from build123d import *

# Parameters (mm, degrees)
SKETCH_1_W          = 52
SKETCH_1_H          = 63
EXTRUDE_1_DEPTH     = 8
SKETCH_2_W          = 48.4
SKETCH_2_H          = 59.4
CUT_EXTRUDE_1_DEPTH = 6.3
FILLET_1_R          = 2
CUT_EXTRUDE_2_REACH = 43.327
SKETCH_3_R          = 3.2
CUT_EXTRUDE_3_REACH = 43.327
SKETCH_4_R          = 18
SKETCH_4_W          = 13.4
SKETCH_4_H          = 3
CUT_EXTRUDE_4_REACH = 43.327
SKETCH_5_W          = 5.3
SKETCH_5_H          = 3.2
SKETCH_6_W          = 10
SKETCH_6_H          = 2.2
SKETCH_6_W_2        = 4.8
SKETCH_6_W_3        = 6.5
SKETCH_6_H_2        = 10
CUT_EXTRUDE_5_DEPTH = 1
CUT_EXTRUDE_6_REACH = 61.802
SKETCH_7_W          = 6.3
SKETCH_7_H          = 10


with BuildPart() as part:
    # 草图1 → 凸台-拉伸1 (new body)
    with BuildSketch(Plane.XY):
        Rectangle(SKETCH_1_W, SKETCH_1_H)
    extrude(amount=EXTRUDE_1_DEPTH)

    # 草图2 → 切除-拉伸1 (cut)
    with BuildSketch(Plane.XY.offset(8)):
        Rectangle(SKETCH_2_W, SKETCH_2_H)
    extrude(amount=-CUT_EXTRUDE_1_DEPTH, mode=Mode.SUBTRACT)

    # 圆角1
    fillet_1_edges = [part.edges().sort_by_distance(p)[0] for p in [
        (26, -31.5, 4),
        (-26, -31.5, 4),
        (-26, 31.5, 4),
        (26, 31.5, 4),
    ]]
    fillet(fillet_1_edges, radius=FILLET_1_R)

    # 草图3 → 切除-拉伸2 (cut, up to next)
    with BuildSketch(Plane.XY.offset(1.7), mode=Mode.PRIVATE) as cut_extrude_2_sk1:
        with Locations((0, 24)):
            Circle(SKETCH_3_R)
    cut_extrude_2_tool1 = extrude(cut_extrude_2_sk1.sketch, amount=-CUT_EXTRUDE_2_REACH, mode=Mode.PRIVATE) & part.part
    # 草图3 → 切除-拉伸2 (cut, up to next)
    with BuildSketch(Plane.XY.offset(1.7), mode=Mode.PRIVATE) as cut_extrude_2_sk2:
        with Locations((-17.8, -24)):
            Circle(SKETCH_3_R)
    cut_extrude_2_tool2 = extrude(cut_extrude_2_sk2.sketch, amount=-CUT_EXTRUDE_2_REACH, mode=Mode.PRIVATE) & part.part
    # 草图3 → 切除-拉伸2 (cut, up to next)
    with BuildSketch(Plane.XY.offset(1.7), mode=Mode.PRIVATE) as cut_extrude_2_sk3:
        with Locations((17.8, -24)):
            Circle(SKETCH_3_R)
    cut_extrude_2_tool3 = extrude(cut_extrude_2_sk3.sketch, amount=-CUT_EXTRUDE_2_REACH, mode=Mode.PRIVATE) & part.part
    add(cut_extrude_2_tool1.solids().sort_by_distance((0, 24, 1.7))[0], mode=Mode.SUBTRACT)
    add(cut_extrude_2_tool2.solids().sort_by_distance((-17.8, -24, 1.7))[0], mode=Mode.SUBTRACT)
    add(cut_extrude_2_tool3.solids().sort_by_distance((17.8, -24, 1.7))[0], mode=Mode.SUBTRACT)

    # 草图4 → 切除-拉伸3 (cut, up to next)
    with BuildSketch(Plane.XY.offset(1.7), mode=Mode.PRIVATE) as cut_extrude_3_sk1:
        Circle(SKETCH_4_R)
    cut_extrude_3_tool1 = extrude(cut_extrude_3_sk1.sketch, amount=-CUT_EXTRUDE_3_REACH, mode=Mode.PRIVATE) & part.part
    # 草图4 → 切除-拉伸3 (cut, up to next)
    with BuildSketch(Plane.XY.offset(1.7), mode=Mode.PRIVATE) as cut_extrude_3_sk2:
        with BuildLine():
            ThreePointArc((7.65, -16.293480291), (0, -18), (-7.65, -16.293480291))
            Line((-7.65, -16.293480291), (-6.7, -19.893480291))
            Line((-6.7, -19.893480291), (6.7, -19.893480291))
            Line((6.7, -19.893480291), (7.65, -16.293480291))
        make_face()
    cut_extrude_3_tool2 = extrude(cut_extrude_3_sk2.sketch, amount=-CUT_EXTRUDE_3_REACH, mode=Mode.PRIVATE) & part.part
    # 草图4 → 切除-拉伸3 (cut, up to next)
    with BuildSketch(Plane.XY.offset(1.7), mode=Mode.PRIVATE) as cut_extrude_3_sk3:
        with Locations((0, -21.393480291)):
            Rectangle(SKETCH_4_W, SKETCH_4_H)
    cut_extrude_3_tool3 = extrude(cut_extrude_3_sk3.sketch, amount=-CUT_EXTRUDE_3_REACH, mode=Mode.PRIVATE) & part.part
    add(cut_extrude_3_tool1.solids().sort_by_distance((0, 0, 1.7))[0], mode=Mode.SUBTRACT)
    add(cut_extrude_3_tool2.solids().sort_by_distance((0, -18.608129, 1.7))[0], mode=Mode.SUBTRACT)
    add(cut_extrude_3_tool3.solids().sort_by_distance((0, -21.39348, 1.7))[0], mode=Mode.SUBTRACT)

    # 草图5 → 切除-拉伸4 (cut, up to next)
    with BuildSketch(Plane.XY.offset(1.7), mode=Mode.PRIVATE) as cut_extrude_4_sk1:
        with Locations((15, 20)):
            Rectangle(SKETCH_5_W, SKETCH_5_H)
    cut_extrude_4_tool1 = extrude(cut_extrude_4_sk1.sketch, amount=-CUT_EXTRUDE_4_REACH, mode=Mode.PRIVATE) & part.part
    add(cut_extrude_4_tool1.solids().sort_by_distance((15, 20, 1.7))[0], mode=Mode.SUBTRACT)

    # 草图6 → 切除-拉伸5 (cut)
    with BuildSketch(Plane.XY.offset(1.7)):
        with Locations((-15, 25)):
            Rectangle(SKETCH_6_W, SKETCH_6_H)
        with Locations((15, 25)):
            Rectangle(SKETCH_6_W, SKETCH_6_H)
        with Locations((17, -15)):
            Rectangle(SKETCH_6_W, SKETCH_6_H)
        with Locations((-13.5, -17.5)):
            Rectangle(SKETCH_6_W_2, SKETCH_6_H)
        with Locations((-19, 16)):
            Rectangle(SKETCH_6_W_3, SKETCH_6_H_2)
    extrude(amount=-CUT_EXTRUDE_5_DEPTH, mode=Mode.SUBTRACT)

    # 草图7 → 切除-拉伸6 (cut, up to next)
    with BuildSketch(Plane(origin=(-24.2, 0, 0), x_dir=(0, 0, -1), z_dir=(1, 0, 0)), mode=Mode.PRIVATE) as cut_extrude_6_sk1:
        with Locations((-4.85, 15.863241886)):
            Rectangle(SKETCH_7_W, SKETCH_7_H)
    cut_extrude_6_tool1 = extrude(cut_extrude_6_sk1.sketch, amount=-CUT_EXTRUDE_6_REACH, mode=Mode.PRIVATE) & part.part
    add(cut_extrude_6_tool1.solids().sort_by_distance((-24.2, 15.863242, 4.85))[0], mode=Mode.SUBTRACT)


solid = part.part
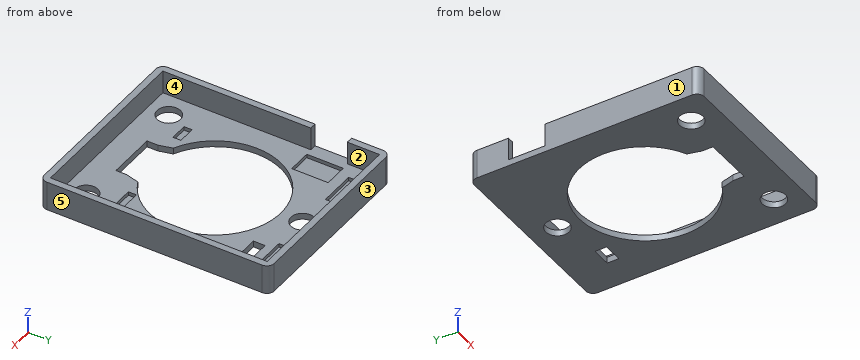
The model under review builds one solid part; all positions refer to its coordinate system, in mm. Face numbers are marked on the shaded views. A direction names the side the tool comes from. Give positions to 0.01 mm unless a question says otherwise; leave off trailing zeros. Order: outer loops, then holes, each group sorted by start corner. A loop starts at its lowest first (then second) coordinate and runs counter-clockwise, first axis right, second up. Notation, with made-up numbers: (87.25, 2.25) -> (122.25, 2.25) arc R31 cw to (122.25, 26.25) -> close; hole circle Ø1 at (73.5, 57.25). An arc over 180 degrees is marked (long way). Write item = value, one per line. Start each with the question number.
(1) For pin 1 Ø4 at (x, y) = (7.5, -13) entering from -Z; pin 2 Ø0.9 at (x, z) = (-25, 5) entering from +Y; pin 3 Ø1.8 at (x, y) = (-14, 25.5) entering from +Z; pin 4 Ø0.7 at (x, y) = (17.5, -15) entering from +Z, all flat-tipped, find the tip position at first contact; note any pin that passes through.
(2) For L1, parallel to Y at x = 0, z = 0.9; L2, parallel to Y at x = -9, z = 4; L3, parallel to X at y = 21.5, z = 5, list the stretches that pass through material, from the lowest coordinate up. Write a range as from..to.
(3) Take a section at D-D (x = -5.5). Write out the cut boundary in (y, z).
(4) Take a section at B-B (y = -24). Write out the cut boundary in (x, z), plus the area to 3 significant figures.
(5) Take a section at A-A (y = 0). Write out the cut boundary in (x, z).
(6) Take a section at C-C (z = 4.5). Write out the cut boundary in (x, y).
(7) Draft analysis for pull direction Y (two halves, no side actions). For the marked faces 1, 2 and 3, state which applies: +Y half, -Y half, draft (parallel to the pull), parting line (faces both ways), or undercut.
(8) Tool access review of the marked faces 4 and 5: name each direction out of +Z, -Z, +X, -X, +Y, -Y from which nothing blocks a thin tool from reaching the whole face with its end or side.
Returned:
q1.pin_1 = through
q1.pin_2 = 31.42
q1.pin_3 = 1.7
q1.pin_4 = 0.7
q2.L1 = -31.5..-22.89, 18..20.8, 27.2..31.5
q2.L2 = -31.5..-29.7, 29.7..31.5
q2.L3 = -26..-24.2, 24.2..26
q3.outline = (-31.5, 0) -> (-22.89, 0) -> (-22.89, 1.7) -> (-29.7, 1.7) -> (-29.7, 8) -> (-31.5, 8) -> close; (17.14, 0) -> (31.5, 0) -> (31.5, 8) -> (29.7, 8) -> (29.7, 1.7) -> (17.14, 1.7) -> close
q4.outline = (-26, 0) -> (-21, 0) -> (-21, 1.7) -> (-24.2, 1.7) -> (-24.2, 8) -> (-26, 8) -> close; (-14.6, 0) -> (14.6, 0) -> (14.6, 1.7) -> (-14.6, 1.7) -> close; (21, 0) -> (26, 0) -> (26, 8) -> (24.2, 8) -> (24.2, 1.7) -> (21, 1.7) -> close
q4.area = 89.3 mm²
q5.outline = (-26, 0) -> (-18, 0) -> (-18, 1.7) -> (-24.2, 1.7) -> (-24.2, 8) -> (-26, 8) -> close; (18, 0) -> (26, 0) -> (26, 8) -> (24.2, 8) -> (24.2, 1.7) -> (18, 1.7) -> close
q6.outline = (-26, -29.5) arc R2 ccw to (-24, -31.5) -> (24, -31.5) arc R2 ccw to (26, -29.5) -> (26, 29.5) arc R2 ccw to (24, 31.5) -> (-24, 31.5) arc R2 ccw to (-26, 29.5) -> (-26, 20.86) -> (-24.2, 20.86) -> (-24.2, 29.7) -> (24.2, 29.7) -> (24.2, -29.7) -> (-24.2, -29.7) -> (-24.2, 10.86) -> (-26, 10.86) -> close
q7.face_1 = draft
q7.face_2 = undercut
q7.face_3 = +Y half
q8.face_4 = +Z
q8.face_5 = +Z, -Z, +X, +Y, -Y
